from build123d import *

# Parameters (mm, degrees)
SKETCH_R     = 12
PAD_DEPTH    = 30
SKETCH001_R  = 3
PAD001_DEPTH = 1
SKETCH002_R  = 1
PAD002_DEPTH = 10
SKETCH003_R  = 1
POCKET_DEPTH = 4


with BuildPart() as part:
    # Sketch → Pad (new body)
    with BuildSketch(Plane.XY):
        Circle(SKETCH_R)
    extrude(amount=PAD_DEPTH)

    # Sketch001 (on Face3 of Pad) → Pad001 (join)
    with BuildSketch(Plane.XY.offset(30)):
        Circle(SKETCH001_R)
    extrude(amount=PAD001_DEPTH)

    # Sketch002 (on Face5 of Pad001) → Pad002 (join)
    with BuildSketch(Plane.XY.offset(31)):
        Circle(SKETCH002_R)
    extrude(amount=PAD002_DEPTH)

    # Sketch003 (on Face3 of Pad002) → Pocket (cut)
    with BuildSketch(Plane.XY.offset(30)):
        with Locations((-7, 0)):
            Circle(SKETCH003_R)
        with Locations((7, 0)):
            Circle(SKETCH003_R)
    extrude(amount=-POCKET_DEPTH, mode=Mode.SUBTRACT)


solid = part.part
CAD build for the part. Positions are in the model's coordinates, mm. A direction names the side the tool comes from. Round coordinates to 2 decimals unless told otherwise and drop trailing zeros. Order: outer loops, then holes, each group sorted by start corner. A loop starts at its lowest first (then second) coordinate and runs counter-clockwise, first axis right, second up. Notation, with made-up numbers: (20.5, -10.75) -> (64.5, -10.75) arc R11 cw to (64.5, -0.75) -> close; hole circle Ø2 at (12, 14). An arc over 180 degrees is marked (long way). Write item = value, one per line. Start each with the question number.
(1) Cut at A-A, the plane y = 0. List the corners of the cut face in (x, z), then the cut area to 3 significant figures.
(2) Which spindle directions (+Z, -Z, +X, -X, +Y, -Y) get a long thin tool onto all of the face, cutting with end or side? Do faces 1 (the flat face through (0, 0, 41)), 2 (the flat face through (7, 0, 26)). Say none if no direction does.
(3) Pull direction X, two halves, no side cores. Call faces 3 (the cylindrical face through (-7.8, -0.6, 28)), 4 (the cylindrical face through (-11.99, 0.53, 14.79)), 5 (the flat face through (0, 0, 0)): released by +X, released by -X, zero draft, split by the parting line, or undercut.
(4) Cut at D-D, the plane x = 7. List the corners of the cut face in (y, z), then the cut area to 3 significant figures.
(5) Probe line 1 (Z direction, x = 3.25, y = 8.5); line 2 (Y direction, x = -7, z = 28.2); line 3 (X direction, y = 0.25, z = 25). List the from-to ranges inside material, lowest first. Write a range as [from, to].
(6) Pin check, flat tips, straight feed: P1, Ø3, axis at x = -7, z = 16, coming from the +Y side; P2, Ø8, axis at x = -5, z = 12, coming from the -Y side; P3, Ø5, axis at y = -7.5, z = 26.5, coming from the +X side. Stop position of each tip, or through.
(7) Cut at C-C, the plane z = 7.5. List the corners of the cut face in (x, y).
(8) Cut at B-B, the plane x = 0. List the corners of the cut face in (y, z).
Model answer:
q1.outline = (-12, 0) -> (12, 0) -> (12, 30) -> (8, 30) -> (8, 26) -> (6, 26) -> (6, 30) -> (3, 30) -> (3, 31) -> (1, 31) -> (1, 41) -> (-1, 41) -> (-1, 31) -> (-3, 31) -> (-3, 30) -> (-6, 30) -> (-6, 26) -> (-8, 26) -> (-8, 30) -> (-12, 30) -> close
q1.area = 730 mm2
q2.face_1 = +Z, +X, -X, +Y, -Y
q2.face_2 = +Z
q3.face_3 = undercut
q3.face_4 = split by the parting line
q3.face_5 = zero draft
q4.outline = (-9.75, 0) -> (9.75, 0) -> (9.75, 30) -> (1, 30) -> (1, 26) -> (-1, 26) -> (-1, 30) -> (-9.75, 30) -> close
q4.area = 577 mm2
q5.line_1 = [0, 30]
q5.line_2 = [-9.75, -1], [1, 9.75]
q5.line_3 = [-12, 12]
q6.P1 = 10.67
q6.P2 = -11.96
q6.P3 = 10.91
q7.outline = circle Ø24 at (0, 0)
q8.outline = (-12, 0) -> (12, 0) -> (12, 30) -> (3, 30) -> (3, 31) -> (1, 31) -> (1, 41) -> (-1, 41) -> (-1, 31) -> (-3, 31) -> (-3, 30) -> (-12, 30) -> close
